from build123d import *

# Parameters (mm, degrees)
SKETCH1_W           = 3
SKETCH1_H           = 9.45
BASE_EXTRUDE_DEPTH  = 3
SKETCH2_W           = 10
SKETCH2_H           = 3
BOSS_EXTRUDE1_DEPTH = 3


with BuildPart() as part:
    # Sketch1 → Base-Extrude (new body)
    with BuildSketch(Plane.XY):
        with BuildLine():
            Line((1079.876919763, -44.105153511), (1068.056216666, -10.172974917))
            Line((1068.056216666, -10.172974917), (1065.157526034, 2.696840543))
            Line((1065.157526034, 2.696840543), (1048.759611565, 48.101577381))
            ThreePointArc((1048.759611565, 48.101577381), (1032.394850119, 46.101647559), (1016.466345621, 41.848662618))
            Line((1016.466345621, 41.848662618), (1016.466345621, 39.392602571))
            Line((1016.466345621, 39.392602571), (1035.726137056, 39.392602571))
            Line((1035.726137056, 39.392602571), (1035.726137056, 36.392602571))
            Line((1035.726137056, 36.392602571), (1009.279499751, 36.392602571))
            Line((1009.279499751, 36.392602571), (1009.279499751, -89.073987735))
            Line((1009.279499751, -89.073987735), (1032.543515661, -98.536722682))
            Line((1032.543515661, -98.536722682), (1040.991113984, -80.770341528))
            Line((1040.991113984, -80.770341528), (1072.440441541, -58.876157059))
            Line((1072.440441541, -58.876157059), (1076.9710582, -54.961956755))
            ThreePointArc((1076.9710582, -54.961956755), (1080.093496996, -49.980404823), (1079.876919763, -44.105153511))
        make_face()
        with BuildLine():
            Line((1019.213878108, 30.925856164), (1019.213878108, 6.018771541))
            Line((1019.213878108, 6.018771541), (1016.100082492, -1.038872257))
            Line((1016.100082492, -1.038872257), (1016.100082492, -55.976738358))
            Line((1016.100082492, -55.976738358), (1019.100082492, -55.976738358))
            Line((1019.100082492, -55.976738358), (1019.100082492, -43.198135443))
            Line((1019.100082492, -43.198135443), (1023.478597046, -41.580404808))
            Line((1023.478597046, -41.580404808), (1023.478597046, -73.992128786))
            Line((1023.478597046, -73.992128786), (1032.526582577, -78.167039678))
            Line((1032.526582577, -78.167039678), (1068.850484509, -50.258348586))
            ThreePointArc((1068.850484509, -50.258348586), (1070.803657728, -46.221334872), (1068.734776871, -42.242378056))
            Line((1068.734776871, -42.242378056), (1063.325122863, -38.329012558))
            Line((1063.325122863, -38.329012558), (1062.407393196, -36.386031272))
            Line((1062.407393196, -36.386031272), (1069.115709638, -34.04910449))
            Line((1069.115709638, -34.04910449), (1062.700744223, -15.634484789))
            Line((1062.700744223, -15.634484789), (1056.810312455, -17.686491112))
            Line((1056.810312455, -17.686491112), (1052.869598475, -15.779326268))
            Line((1052.869598475, -15.779326268), (1050.941521122, -1.083078235))
            Line((1050.941521122, -1.083078235), (1057.625060998, 1.362146575))
            Line((1057.625060998, 1.362146575), (1056.321001716, 4.948397029))
            Line((1056.321001716, 4.948397029), (1046.214175082, 4.948397029))
            Line((1046.214175082, 4.948397029), (1041.773169547, 17.294470752))
            Line((1041.773169547, 17.294470752), (1047.600835278, 23.111994965))
            Line((1047.600835278, 23.111994965), (1051.253809923, 12.605592538))
            Line((1051.253809923, 12.605592538), (1054.100349004, 13.552807012))
            Line((1054.100349004, 13.552807012), (1049.909104568, 25.720739733))
            Line((1049.909104568, 25.720739733), (1046.816291402, 30.939914406))
            Line((1046.816291402, 30.939914406), (1019.213878108, 30.925856164))
        make_face(mode=Mode.SUBTRACT)
        Polygon((1012.307844389, -84.207250741), (1013.438177941, -81.428339792), (1030.025357256, -88.175243766), (1028.895023704, -90.954154714), align=None, mode=Mode.SUBTRACT)
        with Locations((1013.982987836, 18.006853638)):
            Rectangle(SKETCH1_W, SKETCH1_H, mode=Mode.SUBTRACT)
    extrude(amount=BASE_EXTRUDE_DEPTH)

    # Sketch2 → Boss-Extrude1 (add)
    with BuildSketch(Plane.XY.offset(3)):
        with Locations((1030.726137056, 37.892602571)):
            Rectangle(SKETCH2_W, SKETCH2_H)
    extrude(amount=-BOSS_EXTRUDE1_DEPTH)


solid = part.part
For this review, take the finished solid that the model builds, in its own axes (mm). A direction names the side the tool comes from. Coordinates: 2 decimals unless noted, no trailing zeros. Order: outer loops, then holes, each group sorted by start corner. A loop starts at its lowest first (then second) coordinate and runs counter-clockwise, first axis right, second up. Notation, with made-up numbers: (71, 27) - (93, 27) arc R22 ccw to (93, 43) - close; hole circle Ø3 at (55, 71). An arc over 180 degrees is marked (long way). Answer as CSV lines item,"result". Start each with the question number.
1) Machinability: for faces 1 (the flat face through (1049.402, 17.932, 1.479)), 2 (the flat face through (1074.05, -27.38, 1.48)), 3 (the flat face through (1016.466, 41, 1)), which of the approach directions +Z, -Z, +X, -X, +Y, -Y give a long, thin tool a straight path to every point of the face, cutting with its end or side? Answer none if there is none.
2) To check wall thickness, follow line 1 along X through (y, z) = (18, 0.3); line 2 along X through (y, z) = (15, 1.2); line 3 along Y through (x, z) = (1014, 0.3). State the ranges of each line that lie inside material, in increasing order. Write a range as [from, to].
3) Add section D-D (z = 1.2). Count the separate pieces of the cut face and the enclosed holes in it, then the cut area to 3 significant figures.
4) Insertion check: P1, Ø1.5, axis at x = 1021.5, z = 1.5, coming from the -Y side; P2, Ø0.9, axis at x = 1014.5, z = 2, coming from the -Y side. Each pin has a flat end and moves straight along its axis. Give the tip position at first contact, or say it passes through.
5) Add section B-B (y = -63). State the section outline as (x, z) points, then the cut area to 3 significant figures.
6) Add section C-C (x = 1021.5). State the section outline as (y, z) points.
7) Draft analysis for pull direction X (two halves, no side actions). For faces 4 (the flat face through (1021.26, -42.4, 1.48)), 5 (the flat face through (1015.483, 18, 1)), 6 (the cylindrical face through (1080.07, -50.06, 1.48)), 7 (the flat face through (1020.75, -93.74, 1.48)), state which applies: +X half, -X half, draft (parallel to the pull), parting line (faces both ways), or undercut.
8) Add section A-A (x = 1038). State the section outline as (y, z) points.
Result:
1,face 1,"+Z, -Z"
1,face 2,"+Z, -Z, +X, +Y"
1,face 3,"+Z, -Z, -X, +Y"
2,line 1,"[1009.28, 1012.48], [1015.48, 1019.21], [1042.48, 1049.38], [1052.57, 1059.63]"
2,line 2,"[1009.28, 1012.48], [1015.48, 1019.21], [1042.6, 1050.42], [1053.6, 1060.71]"
2,line 3,"[-90.99, -84.9], [-81.66, 13.28], [22.73, 36.39]"
3,separate pieces,"1"
3,enclosed holes,"3"
3,area,"3,330 mm^2"
4,P1,"y = -94.35"
4,P2,"y = -91.38"
5,outline,"(1009.28, 0) - (1023.48, 0) - (1023.48, 3) - (1009.28, 3) - close; (1052.27, 0) - (1066.52, 0) - (1066.52, 3) - (1052.27, 3) - close"
5,area,"85.3 mm^2"
6,outline,"(-94.04, 0) - (-87.95, 0) - (-87.95, 3) - (-94.04, 3) - close; (-84.71, 0) - (-42.31, 0) - (-42.31, 3) - (-84.71, 3) - close; (30.93, 0) - (36.39, 0) - (36.39, 3) - (30.93, 3) - close; (39.39, 0) - (43.45, 0) - (43.45, 3) - (39.39, 3) - close"
7,face 4,"undercut"
7,face 5,"undercut"
7,face 6,"+X half"
7,face 7,"-X half"
8,outline,"(-87.06, 0) - (-73.96, 0) - (-73.96, 3) - (-87.06, 3) - close; (30.94, 0) - (47.05, 0) - (47.05, 3) - (30.94, 3) - close"
